Build history of the part. All positions in model axes, mm. Give positions to 0.01 mm unless a question says otherwise; leave off trailing zeros. Write item = value, one per line. Start each with the question number.
Q1. Wall check: line 1 (Y direction, x = 32.5, z = 46.25); line 2 (X direction, y = 32.5, z = 48.65); line 3 (Y direction, x = 32, z = 48). Give the ranges that are in metal, low to high.
Q2. Mould opens along X. For faces 1 (the face through (0, 58, 25)), 2 (the face through (106, 58, 0)), 3 (the face through (215, 57, 25)) say: pulls with the +X half, pulls with the -X half, needs draft (parallel to the pull), parting line crosses it, or undercut.
Q3. Drop flat-ended pins along their axis: P1, Ø5, axis at x = 32.5, y = 32.5, coming from the +Z side; P2, Ø3, axis at x = 182.5, y = 82.5, coming from the +Z side. Give the stop position or say it passes through.
Autodesk Inventor part; units mm, degrees
ref_plane "YZ Plane" through (0, 0, 0) normal (1, 0, 0) x (0, 1, 0)
ref_plane "XZ Plane" through (0, 0, 0) normal (0, 1, 0) x (-1, 0, 0)
ref_plane "XY Plane" through (0, 0, 0) normal (0, 0, 1) x (1, 0, 0)
sketch "Sketch1" plane through (0, 0, 0) normal (0, 0, 1) x (1, 0, 0)
  line L0 (0, 0) -> (215, 0)
  line L1 (215, 0) -> (215, 115)
  line L2 (215, 115) -> (0, 115)
  line L3 (0, 115) -> (0, 0)
  dimension "d0" = 215
  dimension "d2" = 115
extrude "Extrusion1" add sketch "Sketch1" along normal blind 50
sketch "Sketch2" plane through (0, 0, 50) normal (0, 0, 1) x (1, 0, 0)
  line L0 (215, 0) -> (215, 115)
  line L1 (215, 115) -> (0, 115)
  line L2 (32.5, 82.5) -> (182.5, 82.5)
  line L3 (182.5, 82.5) -> (182.5, 32.5)
  line L4 (182.5, 32.5) -> (32.5, 32.5)
  line L5 (32.5, 32.5) -> (32.5, 82.5)
  point P0 (107.5, 82.5)
  point P1 (107.5, 115)
  point P2 (182.5, 57.5)
  point P3 (215, 57.5)
  dimension "d5" = 150
  dimension "d7" = 50
hole "Hole1" at (32.5, 82.5, 50) at (32.5, 32.5, 50) at (182.5, 32.5, 50) at (182.5, 82.5, 50) direction (0, 0, -1) diameter 3.242 depth 5 tip angle 118
properties part number "power supply"
Report:
q1.line_1 = 0 to 30.88, 34.12 to 80.88, 84.12 to 115
q1.line_2 = 0 to 30.88, 34.12 to 180.88, 184.12 to 215
q1.line_3 = 0 to 30.96, 34.04 to 80.96, 84.04 to 115
q2.face_1 = pulls with the -X half
q2.face_2 = needs draft
q2.face_3 = pulls with the +X half
q3.P1 = 50
q3.P2 = 44.93
